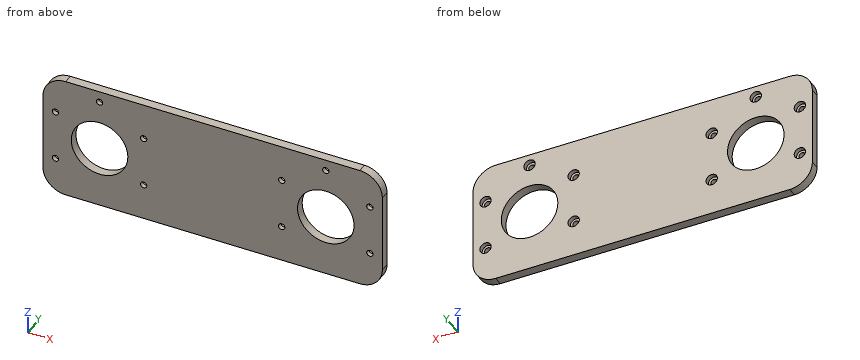
```python
from build123d import *

# Parameters (mm, degrees)
SKETCH1_W           = 150
SKETCH1_H           = 55
SKETCH1_R           = 12.5
BOSS_EXTRUDE1_DEPTH = 4
SKETCH2_R           = 1.4
CUT_EXTRUDE1_DEPTH  = 80.982810653
SKETCH3_R           = 2.5
CUT_EXTRUDE3_DEPTH  = 2
FILLET1_R           = 10


with BuildPart() as part:
    # Sketch1 → Boss-Extrude1 (new body)
    with BuildSketch(Plane(origin=(0, 0, 0), x_dir=(1, 0, 0), z_dir=(0, 1, 0))):
        Rectangle(SKETCH1_W, SKETCH1_H)
        with Locations(Location((-50, 0, 0), (0, 0, 270))):
            Circle(SKETCH1_R, mode=Mode.SUBTRACT)
        with Locations(Location((50, 0, 0), (0, 0, 270))):
            Circle(SKETCH1_R, mode=Mode.SUBTRACT)
    extrude(amount=BOSS_EXTRUDE1_DEPTH)

    # Sketch2 → Cut-Extrude1 (cut, through all)
    with BuildSketch(Plane(origin=(0, 4, 0), x_dir=(1, 0, 0), z_dir=(0, 1, 0))):
        with Locations(Location((30.514428415, 11.25, 0), (0, 0, 270))):
            Circle(SKETCH2_R)
        with Locations(Location((69.485571585, 11.25, 0), (0, 0, 270))):
            Circle(SKETCH2_R)
        with Locations(Location((69.485571585, -11.25, 0), (0, 0, 270))):
            Circle(SKETCH2_R)
        with Locations(Location((30.514428415, -11.25, 0), (0, 0, 270))):
            Circle(SKETCH2_R)
        with Locations(Location((50, -22.5, 0), (0, 0, 270))):
            Circle(SKETCH2_R)
    cut_extrude1 = extrude(amount=-CUT_EXTRUDE1_DEPTH, mode=Mode.SUBTRACT)

    # Sketch3 → Cut-Extrude3 (cut)
    with BuildSketch(Plane(origin=(0, 4, 0), x_dir=(1, 0, 0), z_dir=(0, 1, 0))):
        with Locations(Location((30.514428415, 11.25, 0), (0, 0, 270))):
            Circle(SKETCH3_R)
        with Locations(Location((30.514428415, -11.25, 0), (0, 0, 270))):
            Circle(SKETCH3_R)
        with Locations(Location((50, -22.5, 0), (0, 0, 270))):
            Circle(SKETCH3_R)
        with Locations(Location((69.485571585, -11.25, 0), (0, 0, 270))):
            Circle(SKETCH3_R)
        with Locations(Location((69.485571585, 11.25, 0), (0, 0, 270))):
            Circle(SKETCH3_R)
    cut_extrude3 = extrude(amount=-CUT_EXTRUDE3_DEPTH, mode=Mode.SUBTRACT)

    # Mirror1: Cut-Extrude1, Cut-Extrude3 across plane
    add(cut_extrude1.mirror(Plane(origin=(0, 0, 0), x_dir=(0, 0, 1), z_dir=(1, 0, 0))), mode=Mode.SUBTRACT)
    add(cut_extrude3.mirror(Plane(origin=(0, 0, 0), x_dir=(0, 0, 1), z_dir=(1, 0, 0))), mode=Mode.SUBTRACT)

    # Fillet1
    fillet1_edges = [part.edges().sort_by_distance(p)[0] for p in [
        (-75, 2, -27.5),
        (75, 2, -27.5),
        (75, 2, 27.5),
        (-75, 2, 27.5),
    ]]
    fillet(fillet1_edges, radius=FILLET1_R)


solid = part.part
```
Here's how the part is built. I have some questions about the finished solid (model axes, mm). Coordinates: 2 decimals unless noted, no trailing zeros. Order: outer loops, then holes, each group sorted by start corner. A loop starts at its lowest first (then second) coordinate and runs counter-clockwise, first axis right, second up. Notation, with made-up numbers: M 7.25,43 L 53.25,43 A32 ccw 53.25,78 Z; hole C 58.5,1.25 d9. An arc over 180 degrees is marked long. Answer as a JSON object with one key per item and string values. Group by question number.
(1) For pin 1 (3 mm diameter, centred on x = 30.51, z = 11.25, fed in from +Y), with a flat end and sliding along its axis, tell me the tip position at first contact or that it passes through.
(2) Suppose I cut it at A-A, the plane z = 0. Please give me the cut outline in (x, y).
(3) I need wall thicknesses on probe 1 along X at (y, z) = (3.1, 7); probe 2 along X at (y, z) = (2.7, 21); probe 3 along X at (y, z) = (2.6, -13). Which ranges of each line are inside material? Lowest first, please.
(4) Suppose I cut it at D-D, the plane z = 22.5. Please give me the cut outline in (x, y), then the cut area to 3 significant figures.
(5) Suppose I cut it at C-C, the plane y = 1.35. State how many separate pieces and enclosed holes the cut face has, then the cut area to 3 significant figures.
(6) Suppose I cut it at B-B, the plane x = -58. Please give me the cut outline in (y, z), then the cut area to 3 significant figures.
Values found:
{
 "1": {"pin 1": "stops at y = 2"},
 "2": {"outline": "M -75,0 L -62.5,0 L -62.5,4 L -75,4 Z; M -37.5,0 L 37.5,0 L 37.5,4 L -37.5,4 Z; M 62.5,0 L 75,0 L 75,4 L 62.5,4 Z"},
 "3": {"probe 1": "x = -75 to -60.36, -39.64 to 39.64, 60.36 to 75", "probe 2": "x = -74.37 to -52, -48 to 48, 52 to 74.37", "probe 3": "x = -75 to -71.27, -67.7 to -32.3, -28.73 to 28.73, 32.3 to 67.7, 71.27 to 75"},
 "4": {"outline": "M -73.66,0 L -51.4,0 L -51.4,2 L -52.5,2 L -52.5,4 L -73.66,4 Z; M -48.6,0 L 48.6,0 L 48.6,2 L 47.5,2 L 47.5,4 L -47.5,4 L -47.5,2 L -48.6,2 Z; M 51.4,0 L 73.66,0 L 73.66,4 L 52.5,4 L 52.5,2 L 51.4,2 Z", "area": "558 mm^2"},
 "5": {"separate pieces": "1", "enclosed holes": "12", "area": "7,120 mm^2"},
 "6": {"outline": "M 0,-27.5 L 4,-27.5 L 4,-9.6 L 0,-9.6 Z; M 0,9.6 L 4,9.6 L 4,27.5 L 0,27.5 Z", "area": "143 mm^2"}
}
